Verification items for this drawing (mm, ordinates from the low corner). Round coordinates to 2 decimals unless told otherwise and drop trailing zeros. Order: outer loops, then holes, each group sorted by start corner. A loop starts at its lowest first (then second) coordinate and runs counter-clockwise, first axis right, second up. Notation, with made-up numbers: (72.5, 54) -> (131.5, 54) arc R29 cw to (131.5, 90) -> close; hole circle Ø5 at (70.25, 42). An arc over 180 degrees is marked (long way). Answer in a Markdown table with one row per item. Add a question column.
1. Depth check by flat-ended pin: P1, Ø3, axis at y = 3.5, z = 16, coming from the +X side; P2, Ø2, axis at x = 8, z = 18.5, coming from the +Y side; P3, Ø1.6, axis at x = 45, z = 16.5, coming from the +Y side. Enter the tip coordinate at first touch or a pass-through.
2. Sectioned sample at A-A, the plane y = 3.5. Record the boundary of the cut face in (x, z).
3. Sectioned sample at B-B, the plane z = 36.75. Record the boundary of the cut face in (x, y), then the cut area to 3 significant figures.
4. Material ranges on L1, parallel to Y at x = 15.5, z = 33; L2, parallel to Y at x = 45, z = 25.5, recorded low to high. Write a range as from..to.
5. Draft check along Z on the marked faces 1 and 2. Enter one of: +Z half, -Z half, draft (parallel to the pull), parting line (faces both ways), or undercut.
6. Sectioned sample at C-C, the plane x = 48.75. Record the boundary of the cut face in (y, z).
7. Sectioned sample at D-D, the plane y = 6.5. Record the boundary of the cut face in (x, z), then the cut area to 3 significant figures.
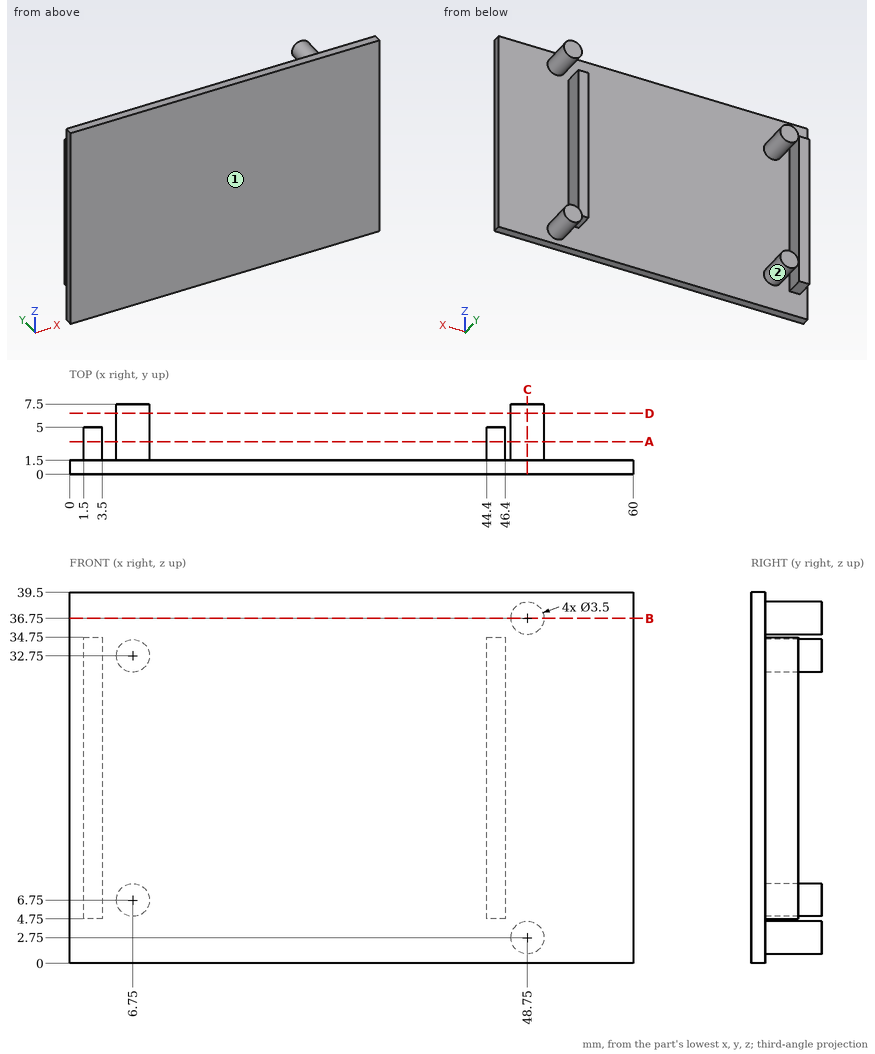
Answer key:
| question | item | result |
|---|---|---|
| 1 | P1 | stops at x = 46.4 |
| 1 | P2 | stops at y = 1.5 |
| 1 | P3 | stops at y = 5 |
| 2 | outline | (1.5, 4.75) -> (3.5, 4.75) -> (3.5, 34.75) -> (1.5, 34.75) -> close; circle Ø3.5 at (6.75, 6.75); circle Ø3.5 at (6.75, 32.75); (44.4, 4.75) -> (46.4, 4.75) -> (46.4, 34.75) -> (44.4, 34.75) -> close; circle Ø3.5 at (48.75, 2.75); circle Ø3.5 at (48.75, 36.75) |
| 3 | outline | (0, 0) -> (60, 0) -> (60, 1.5) -> (50.5, 1.5) -> (50.5, 7.5) -> (47, 7.5) -> (47, 1.5) -> (0, 1.5) -> close |
| 3 | area | 111 mm² |
| 4 | L1 | y = 0..1.5 |
| 4 | L2 | y = 0..5 |
| 5 | face 1 | draft |
| 5 | face 2 | undercut |
| 6 | outline | (0, 0) -> (1.5, 0) -> (1.5, 1) -> (7.5, 1) -> (7.5, 4.5) -> (1.5, 4.5) -> (1.5, 35) -> (7.5, 35) -> (7.5, 38.5) -> (1.5, 38.5) -> (1.5, 39.5) -> (0, 39.5) -> close |
| 7 | outline | circle Ø3.5 at (6.75, 6.75); circle Ø3.5 at (6.75, 32.75); circle Ø3.5 at (48.75, 2.75); circle Ø3.5 at (48.75, 36.75) |
| 7 | area | 38.5 mm² |
